Design review of the part shown in the three views and the two pictorial views. Dimensions are in mm from the part's minimum x, y and z. Coordinates: 2 decimals unless noted, no trailing zeros. Loops run counter-clockwise (first coordinate to the right, second up) from the corner with the lowest first, then second, coordinate; pieces in that order, holes last. Notation, with made-up numbers: (86.5, 13.5) -> (136.5, 13.5) arc R27 ccw to (136.5, 32.5) -> close; hole circle Ø7 at (-11, -30.5). An arc over 180 degrees is marked (long way). One line per item, written item: value.
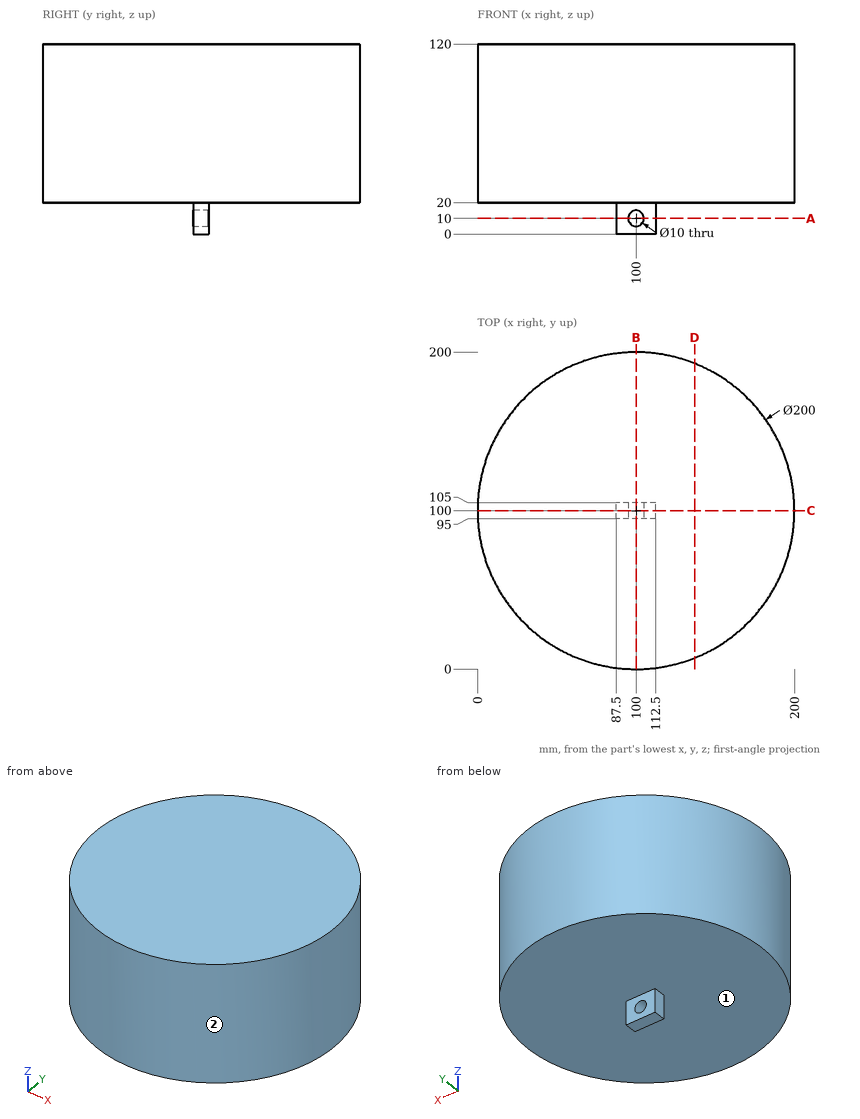
1. To check wall thickness, follow probe 1 along X at (y, z) = (101, 10); probe 2 along Z at (x, y) = (123, 73.5); probe 3 along Y at (x, z) = (140, 105.5). State the ranges of each line that lie inside material, in increasing order. Write a range as from..to.
Return value:
probe 1: x = 87.5..95, 105..112.5
probe 2: z = 20..120
probe 3: y = 8.35..191.65
2. Take a section at A-A, the plane z = 10. Give the boundary of the cut face in (x, y).
Return value:
outline: (87.5, 95) -> (95, 95) -> (95, 105) -> (87.5, 105) -> close; (105, 95) -> (112.5, 95) -> (112.5, 105) -> (105, 105) -> close
3. Take a section at D-D, the plane x = 137. Give the boundary of the cut face in (y, z), and give its area (3 significant figures).
Return value:
outline: (7.1, 20) -> (192.9, 20) -> (192.9, 120) -> (7.1, 120) -> close
area: 18,600 mm2
4. Take a section at B-B, the plane x = 100. Give the boundary of the cut face in (y, z).
Return value:
outline: (0, 20) -> (95, 20) -> (95, 15) -> (105, 15) -> (105, 20) -> (200, 20) -> (200, 120) -> (0, 120) -> close; (95, 0) -> (105, 0) -> (105, 5) -> (95, 5) -> close
5. Insertion check: pin 1 Ø3 at (x, y) = (73, 176.5) entering from -Z; pin 2 Ø8 at (y, z) = (100.5, 14.5) entering from -X; pin 3 Ø5 at (y, z) = (72.5, 17) entering from -X; pin 4 Ø1 at (x, z) = (119.5, 49.5) entering from -Y. Each pin has a flat end and moves straight along its axis. Give the tip position at first contact, or say it passes through.
Return value:
pin 1: stops at z = 20
pin 2: stops at x = 87.5
pin 3: passes through
pin 4: stops at y = 1.82
6. The part is to be moulded in two halves that separate along X. For the marked faces 1 and 2, say which applies: pulls with the +X half, pulls with the -X half, needs draft (parallel to the pull), parting line crosses it, or undercut.
Return value:
face 1: needs draft
face 2: parting line crosses it
7. Take a section at C-C, the plane y = 100. Give the boundary of the cut face in (x, z), and give its area (3 significant figures).
Return value:
outline: (0, 20) -> (87.5, 20) -> (87.5, 0) -> (112.5, 0) -> (112.5, 20) -> (200, 20) -> (200, 120) -> (0, 120) -> close; hole circle Ø10 at (100, 10)
area: 20,400 mm2
